from build123d import *

# Parameters (mm, degrees)
BOSS_EXTRUDE2_DEPTH      = 141
BOSS_EXTRUDE2_DEPTH_BACK = 141
CAVITY1_START            = -323.284735655
CAVITY1_OUTLINE_W        = 282
CAVITY1_OUTLINE_H        = 40
CAVITY1_DEPTH            = 2


# Read off the part's stored shape, not the designer's step: Cavity1
with BuildPart() as part:
    # Sketch1 → Boss-Extrude2 (new, two sides: drawn at the far end of the back side and taken through both)
    with BuildSketch(Plane(origin=(0, 0, -321.284735655), x_dir=(0, 0, -1), z_dir=(1, 0, 0)).offset(-BOSS_EXTRUDE2_DEPTH_BACK)):
        with BuildLine():
            Line((-10, -285), (12, -285))
            Line((12, -285), (12, -330.531793911))
            ThreePointArc((12, -330.531793911), (10.917125793, -335.057815078), (7.903026481, -338.603613927))
            Line((7.903026481, -338.603613927), (-24.863055291, -361.546671381))
            Line((-24.863055291, -361.546671381), (-29.450107081, -354.994945144))
            Line((-29.450107081, -354.994945144), (-4.875892155, -337.787894608))
            Line((-4.875892155, -337.787894608), (-6.023045028, -336.149590519))
            Line((-6.023045028, -336.149590519), (-30.597606357, -353.35688361))
            Line((-30.597606357, -353.35688361), (-34.795346904, -347.361888815))
            Line((-34.795346904, -347.361888815), (-14.264235636, -332.985849937))
            ThreePointArc((-14.264235636, -332.985849937), (-11.129891668, -329.411815627), (-10, -324.794329494))
            Line((-10, -324.794329494), (-10, -285))
        make_face()
    extrude(amount=BOSS_EXTRUDE2_DEPTH + BOSS_EXTRUDE2_DEPTH_BACK)

    # Cavity1 outline → Cavity1 (cut)
    with BuildSketch(Plane.XY.offset(CAVITY1_START)):
        with Locations((0, -305)):
            Rectangle(CAVITY1_OUTLINE_W, CAVITY1_OUTLINE_H)
    extrude(amount=CAVITY1_DEPTH, mode=Mode.SUBTRACT)


solid = part.part
Can you work these out from the model? Positions are in its coordinate system, mm. A direction names the side the tool comes from. Round coordinates to 2 decimals unless told otherwise and drop trailing zeros. Write each loop counter-clockwise with the first axis right and the second up, starting at its lowest first coordinate (ties: lowest second). Pieces come first, ordered by that corner, then holes. Notation, with made-up numbers: M 24.5,3.5 L 49.5,3.5 A24 cw 49.5,33.5 Z; hole C 33.25,-16 d4. An arc over 180 degrees is marked long. Use CSV: the item, a comma, the result in double quotes.
(1) Imagine slicing it at C-C (x = 37). Write out the boundary of the cut face in (y, z).
Check values:
outline,"M -361.55,-296.42 L -338.6,-329.19 A10 ccw -330.53,-333.28 L -285,-333.28 L -285,-323.28 L -325,-323.28 L -325,-321.28 L -285,-321.28 L -285,-311.28 L -324.79,-311.28 A10 cw -332.99,-307.02 L -347.36,-286.49 L -353.36,-290.69 L -336.15,-315.26 L -337.79,-316.41 L -354.99,-291.83 Z"
(2) On a 3-axis mill with a long thin cutter (end or side, diameter ignored), from which of +Z, -Z, +X, -X, +Y, -Y can I reach the whole of each face in a straight line? I mean faces 5 (the flat face through (-2, -305, -321.285)), 6 (the flat face through (-1.97, -344.63, -303.15)), 7 (the flat face through (-2, -305, -311.285)). Say none if no direction works.
Check values:
face 5,"+X, -X, +Y"
face 6,"+X, -X"
face 7,"+Z, +X, -X, +Y"
(3) Imagine slicing it at A-A (y = -316). Write out the boundary of the cut face in (x, z).
Check values:
outline,"M -141,-333.28 L 141,-333.28 L 141,-323.28 L -141,-323.28 Z; M -141,-321.28 L 141,-321.28 L 141,-311.28 L -141,-311.28 Z"
(4) Imagine slicing it at B-B (z = -303). Write out the boundary of the cut face in (x, y).
Check values:
outline,"M -141,-356.94 L 141,-356.94 L 141,-347.18 L -141,-347.18 Z; M -141,-344.74 L 141,-344.74 L 141,-335.8 L -141,-335.8 Z"
(5) We'd pull the mould along Y, two halves only. Please class faces 1 (the flat face through (-1.974, -358.317, -294.16)), 2 (the flat face through (-2, -285, -316)), 3 (the flat face through (-2, -305, -323.285)), 4 (the flat face through (-1.97, -346.51, -303.95)): +Y half, -Y half, draft (parallel to the pull), parting line (faces both ways), or undercut.
Check values:
face 1,"-Y half"
face 2,"+Y half"
face 3,"draft"
face 4,"undercut"
(6) I need wall thicknesses on line 1 along Z through (x, y) = (-118, -324.5); line 2 along Y through (x, z) = (-45, -310); line 3 along Y through (x, z) = (-43, -303.5). Which ranges of each line are inside material? Lowest first, please.
Check values:
line 1,"-333.28 to -323.28, -321.28 to -311.28"
line 2,"-352.04 to -342.28, -339.83 to -329.7"
line 3,"-356.59 to -346.83, -344.39 to -335.45"
(7) I'm going to push flat-ended pins straight in: pin 1 (6 mm diameter, centred on y = -331, z = -307.5, fed in from -X); pin 2 (10 mm diameter, centred on x = -70.5, z = -296, fed in from +Y); pin 3 (12 mm diameter, centred on x = 101.5, z = -327, fed in from -Y); pin 4 (1.5 mm diameter, centred on x = 18, y = -349.5, fed in from -Z). Where does each tip first touch, or does it pass through?
Check values:
pin 1,"x = -141"
pin 2,"y = -337.2"
pin 3,"y = -344.34"
pin 4,"z = -314.7"
